```python
from build123d import *

# Parameters (mm, degrees)
F0_W      = 13.8
F0_H      = 13.8
F1_DEPTH  = 4.5
F2_R      = 6
F3_DEPTH  = 13
F4_R      = 6.45
F5_DEPTH  = 13
F6_R      = 1.5
F7_DEPTH  = 13.801
F9_DEPTH  = 22.001
F10_W     = 6
F10_H     = 6
F11_DEPTH = 6.5
F13_DEPTH = 6.5


with BuildPart() as f1:
    # F0 (on Top) → F1 (new body, symmetric)
    with BuildSketch(Plane.XY):
        Rectangle(F0_W, F0_H)
    extrude(amount=F1_DEPTH, both=True)

    # F2 (on face) → F3 (join)
    with BuildSketch(Plane.XY.offset(4.5)):
        Circle(F2_R)
    extrude(amount=F3_DEPTH)

    # F4 (on face) → F5 (join)
    with BuildSketch(Plane(origin=(0, 0, -4.5), x_dir=(1, 0, 0), z_dir=(0, 0, -1))):
        Circle(F4_R)
    extrude(amount=F5_DEPTH)

    # F6 (on face) → F7 (cut, through all)
    with BuildSketch(Plane.YZ.offset(6.9)):
        Circle(F6_R)
    extrude(amount=-F7_DEPTH, mode=Mode.SUBTRACT)

    # F8 (on face) → F9 (cut, through all)
    with BuildSketch(Plane(origin=(0, 0, -4.5), x_dir=(1, 0, 0), z_dir=(0, 0, -1))):
        Polygon((6.9, 0.8288529099), (6.3405334204, 0), (6.9, -0.8288529099), align=None)
        Polygon((-6.9, -0.7952927344), (-6.2937744095, 0), (-6.9, 0.7952927344), align=None)
    extrude(amount=-F9_DEPTH, mode=Mode.SUBTRACT)

    # F10 (on face) → F11 (cut)
    with BuildSketch(Plane.XY.offset(17.5)):
        Rectangle(F10_W, F10_H)
    extrude(amount=-F11_DEPTH, mode=Mode.SUBTRACT)

    # F12 (on face) → F13 (cut)
    with BuildSketch(Plane(origin=(0, 0, -17.5), x_dir=(1, 0, 0), z_dir=(0, 0, -1))):
        with BuildLine():
            ThreePointArc((3.5496478699, -2.15), (3.9970951114, -1.1161230533), (4.15, 0))
            ThreePointArc((4.15, 0), (-1.1161230533, 3.9970951114), (-3.5496478699, -2.15))
            Line((-3.5496478699, -2.15), (0, -2.15))
            Line((0, -2.15), (3.5496478699, -2.15))
        make_face()
    extrude(amount=-F13_DEPTH, mode=Mode.SUBTRACT)


solid = f1.part
```
CAD build for the part. Positions are in the model's coordinates, mm. A direction names the side the tool comes from. Coordinates: 2 decimals unless noted, no trailing zeros. Order: outer loops, then holes, each group sorted by start corner. A loop starts at its lowest first (then second) coordinate and runs counter-clockwise, first axis right, second up. Notation, with made-up numbers: (81.5, 35.5) - (110.5, 35.5) arc R26 ccw to (110.5, 67.5) - close; hole circle Ø7 at (-15, 32.25). An arc over 180 degrees is marked (long way). Use a Markdown table: item, result. Add a question column.
(1) Drill centre lines: line 1 along X through (y, z) = (0, -12.25); line 2 along Z through (x, y) = (-3.25, 0); line 3 along Y through (x, z) = (2.25, 13). Where is each one in solid material? Low to high. Write a range as [from, to].
(2) Saw through at B-B (z = 0). Give the cut face in (x, y), then the cut area to 3 significant figures.
(3) Flat gauge pins, fed straight in: pin 1 (1.5 mm diameter, centred on x = -1, z = -10, fed in from +Y); pin 2 (3 mm diameter, centred on y = 0, z = 15.5, fed in from -X); pin 3 (6.5 mm diameter, centred on x = 1, z = 14, fed in from +Y). Where does each tip first touch, or does it go through?
(4) Pull direction X, two halves, no side cores. Call faces 1 (the face through (0, 3, 14)), 2 (the face through (6.9, -4, 0)), 3 (the face through (0.1, -1.5, 0.07)): +X half, -X half, draft (parallel to the pull), parting line (faces both ways), or undercut.
(5) Which spindle directions (+Z, -Z, +X, -X, +Y, -Y) get a long thin tool onto all of the face, cutting with end or side? Do faces 4 (the face through (0, -4, 17.5)), 5 (the face through (0, -3, 14)), 6 (the face through (-1.398, 6.297, -10.909)), 7 (the face through (6.624, -0.42, 2.852)), 8 (the face through (6.9, 4, 0)). Say none if no direction does.
(6) Saw through at C-C (z = -14.5). Give the cut face in (x, y).
(7) Saw through at D-D (y = 2.5). Give the cut face in (x, z), then the cut area to 3 significant figures.
(8) Saw through at A-A (x = 0). Give the cut face in (y, z), then the cut area to 3 significant figures.
Solved:
| question | item | result |
|---|---|---|
| 1 | line 1 | x = [-6.45, -4.15], [4.15, 6.45] |
| 1 | line 2 | z = [-11, -1.5], [1.5, 17.5] |
| 1 | line 3 | y = [-5.56, -3], [3, 5.56] |
| 2 | outline | (-6.9, -6.9) - (6.9, -6.9) - (6.9, -1.5) - (-6.9, -1.5) - close; (-6.9, 1.5) - (6.9, 1.5) - (6.9, 6.9) - (-6.9, 6.9) - close |
| 2 | area | 149 mm² |
| 3 | pin 1 | stops at y = 6.45 |
| 3 | pin 2 | stops at x = -6 |
| 3 | pin 3 | stops at y = 6 |
| 4 | face 1 | undercut |
| 4 | face 2 | +X half |
| 4 | face 3 | draft |
| 5 | face 4 | +Z, +X, -X, +Y, -Y |
| 5 | face 5 | +Z |
| 5 | face 6 | -Z |
| 5 | face 7 | +Z, +X |
| 5 | face 8 | +Z, -Z, +X, +Y, -Y |
| 6 | outline | circle Ø12.9 at (0, 0); hole (-3.55, 2.15) arc R4.15 ccw (long way) to (3.55, 2.15) - close |
| 7 | outline | (-6.9, -4.5) - (-5.95, -4.5) - (-5.95, -17.5) - (5.95, -17.5) - (5.95, -4.5) - (6.9, -4.5) - (6.9, 4.5) - (5.45, 4.5) - (5.45, 17.5) - (3, 17.5) - (3, 11) - (-3, 11) - (-3, 17.5) - (-5.45, 17.5) - (-5.45, 4.5) - (-6.9, 4.5) - close |
| 7 | area | 382 mm² |
| 8 | outline | (-6.9, -4.5) - (-6.45, -4.5) - (-6.45, -17.5) - (-4.15, -17.5) - (-4.15, -11) - (2.15, -11) - (2.15, -17.5) - (6.45, -17.5) - (6.45, -4.5) - (6.9, -4.5) - (6.9, 4.5) - (6, 4.5) - (6, 17.5) - (3, 17.5) - (3, 11) - (-3, 11) - (-3, 17.5) - (-6, 17.5) - (-6, 4.5) - (-6.9, 4.5) - close; hole circle Ø3 at (0, 0) |
| 8 | area | 361 mm² |
